Design review of the part built by this model. Coordinates are the model's own, in mm. Give positions to 0.01 mm unless a question says otherwise; leave off trailing zeros. Write each loop counter-clockwise with the first axis right and the second up, starting at its lowest first coordinate (ties: lowest second). Pieces come first, ordered by that corner, then holes. Notation, with made-up numbers: M 84.5,89.25 L 99.5,89.25 A12 ccw 99.5,93.25 Z; hole C 72,84.5 d3. An arc over 180 degrees is marked long. Answer in a Markdown table with one row per item.
```python
from build123d import *

# Parameters (mm, degrees)
F0_W     = 120
F0_H     = 67.5
F0_W_2   = 110.000002
F0_H_2   = 57.500002
F1_DEPTH = 4
F2_W     = 110.000002
F2_H     = 57.500002
F3_DEPTH = 0.2


with BuildPart() as f1:
    # F0 (on Top) → F1 (new body)
    with BuildSketch(Plane.XY):
        Rectangle(F0_W, F0_H)
        Rectangle(F0_W_2, F0_H_2, mode=Mode.SUBTRACT)
        Rectangle(F0_W_2, F0_H_2)
    extrude(amount=F1_DEPTH)

    # F2 (on face) → F3 (cut)
    with BuildSketch(Plane.XY.offset(4)):
        Rectangle(F2_W, F2_H)
    extrude(amount=-F3_DEPTH, mode=Mode.SUBTRACT)


solid = f1.part
```
1) Insertion check: P1, Ø1.5, axis at x = -1.5, y = -17, coming from the +Z side; P2, Ø3, axis at x = 41, y = 17, coming from the -Z side. Each pin has a flat end and moves straight along its axis. Give the tip position at first contact, or say it passes through.
Geometry says:
| item | result |
|---|---|
| P1 | z = 3.8 |
| P2 | z = 0 |
2) Add section B-B (y = -25.5). Write out the cut boundary in (x, z), and give its area (3 significant figures).
Geometry says:
| item | result |
|---|---|
| outline | M -60,0 L 60,0 L 60,4 L 55,4 L 55,3.8 L -55,3.8 L -55,4 L -60,4 Z |
| area | 458 mm^2 |
3) The part is to be moulded in two halves that separate along Y. For faces 1 (the face through (-1, 0, 0)), 2 (the face through (-1, -33.75, 2)), 3 (the face through (-1, 0, 3.8)), 4 (the face through (-1, 33.75, 2)), say which applies: released by +Y, released by -Y, zero draft, split by the parting line, or undercut.
Geometry says:
| item | result |
|---|---|
| face 1 | zero draft |
| face 2 | released by -Y |
| face 3 | undercut |
| face 4 | released by +Y |
4) Add section A-A (x = -42). Write out the cut boundary in (y, z).
Geometry says:
| item | result |
|---|---|
| outline | M -33.75,0 L 33.75,0 L 33.75,4 L 28.75,4 L 28.75,3.8 L -28.75,3.8 L -28.75,4 L -33.75,4 Z |
5) To check wall thickness, follow probe 1 along Z at (x, y) = (-30, 6.5). State the ranges of the line that lie inside material, in increasing order. Write a range as [from, to].
Geometry says:
| item | result |
|---|---|
| probe 1 | [0, 3.8] |
